```python
from build123d import *

# Parameters (mm, degrees)
SKETCH1_W           = 28.5
SKETCH1_H           = 25
BOSS_EXTRUDE1_DEPTH = 2
SKETCH2_W           = 28.5
SKETCH2_H           = 25
SKETCH2_W_2         = 25.5
SKETCH2_H_2         = 22
BOSS_EXTRUDE2_DEPTH = 10
SKETCH3_W           = 1.5
SKETCH3_H           = 7
CUT_EXTRUDE1_DEPTH  = 10
SKETCH4_W           = 1.5
SKETCH4_H           = 2.5
CUT_EXTRUDE2_DEPTH  = 6
BOSS_EXTRUDE3_DEPTH = 12
CUT_EXTRUDE3_REACH  = 27.348
SKETCH6_R           = 1.75
FILLET1_R           = 1


with BuildPart() as part:
    # Sketch1 → Boss-Extrude1 (new body)
    with BuildSketch(Plane(origin=(0, 0, 0), x_dir=(1, 0, 0), z_dir=(0, 1, 0))):
        Rectangle(SKETCH1_W, SKETCH1_H)
        with BuildLine():
            Line((-9.25, 5), (9.25, 5))
            ThreePointArc((9.25, 5), (9.780330086, 5.219669914), (10, 5.75))
            Line((10, 5.75), (10, 6.25))
            ThreePointArc((10, 6.25), (9.780330086, 6.780330086), (9.25, 7))
            Line((9.25, 7), (-9.25, 7))
            ThreePointArc((-9.25, 7), (-9.780330086, 6.780330086), (-10, 6.25))
            Line((-10, 6.25), (-10, 5.75))
            ThreePointArc((-10, 5.75), (-9.780330086, 5.219669914), (-9.25, 5))
        make_face(mode=Mode.SUBTRACT)
        with BuildLine():
            Line((-9.25, 4), (9.25, 4))
            ThreePointArc((9.25, 4), (9.780330086, 3.780330086), (10, 3.25))
            Line((10, 3.25), (10, 2.75))
            ThreePointArc((10, 2.75), (9.780330086, 2.219669914), (9.25, 2))
            Line((9.25, 2), (-9.25, 2))
            ThreePointArc((-9.25, 2), (-9.780330086, 2.219669914), (-10, 2.75))
            Line((-10, 2.75), (-10, 3.25))
            ThreePointArc((-10, 3.25), (-9.780330086, 3.780330086), (-9.25, 4))
        make_face(mode=Mode.SUBTRACT)
        with BuildLine():
            Line((-9.25, 8), (9.25, 8))
            ThreePointArc((9.25, 8), (9.780330086, 8.219669914), (10, 8.75))
            Line((10, 8.75), (10, 9.25))
            ThreePointArc((10, 9.25), (9.780330086, 9.780330086), (9.25, 10))
            Line((9.25, 10), (-9.25, 10))
            ThreePointArc((-9.25, 10), (-9.780330086, 9.780330086), (-10, 9.25))
            Line((-10, 9.25), (-10, 8.75))
            ThreePointArc((-10, 8.75), (-9.780330086, 8.219669914), (-9.25, 8))
        make_face(mode=Mode.SUBTRACT)
        with BuildLine():
            Line((10, -9.25), (10, -8.75))
            ThreePointArc((10, -8.75), (9.780330086, -8.219669914), (9.25, -8))
            Line((9.25, -8), (-9.25, -8))
            ThreePointArc((-9.25, -8), (-9.780330086, -8.219669914), (-10, -8.75))
            Line((-10, -8.75), (-10, -9.25))
            ThreePointArc((-10, -9.25), (-9.780330086, -9.780330086), (-9.25, -10))
            Line((-9.25, -10), (9.25, -10))
            ThreePointArc((9.25, -10), (9.780330086, -9.780330086), (10, -9.25))
        make_face(mode=Mode.SUBTRACT)
        with BuildLine():
            Line((10, -6.25), (10, -5.75))
            ThreePointArc((10, -5.75), (9.780330086, -5.219669914), (9.25, -5))
            Line((9.25, -5), (-9.25, -5))
            ThreePointArc((-9.25, -5), (-9.780330086, -5.219669914), (-10, -5.75))
            Line((-10, -5.75), (-10, -6.25))
            ThreePointArc((-10, -6.25), (-9.780330086, -6.780330086), (-9.25, -7))
            Line((-9.25, -7), (9.25, -7))
            ThreePointArc((9.25, -7), (9.780330086, -6.780330086), (10, -6.25))
        make_face(mode=Mode.SUBTRACT)
        with BuildLine():
            Line((10, -3.25), (10, -2.75))
            ThreePointArc((10, -2.75), (9.780330086, -2.219669914), (9.25, -2))
            Line((9.25, -2), (-9.25, -2))
            ThreePointArc((-9.25, -2), (-9.780330086, -2.219669914), (-10, -2.75))
            Line((-10, -2.75), (-10, -3.25))
            ThreePointArc((-10, -3.25), (-9.780330086, -3.780330086), (-9.25, -4))
            Line((-9.25, -4), (9.25, -4))
            ThreePointArc((9.25, -4), (9.780330086, -3.780330086), (10, -3.25))
        make_face(mode=Mode.SUBTRACT)
        with BuildLine():
            Line((-10, 0.25), (-10, -0.25))
            ThreePointArc((-10, -0.25), (-9.780330086, -0.780330086), (-9.25, -1))
            Line((-9.25, -1), (9.25, -1))
            ThreePointArc((9.25, -1), (9.780330086, -0.780330086), (10, -0.25))
            Line((10, -0.25), (10, 0.25))
            ThreePointArc((10, 0.25), (9.780330086, 0.780330086), (9.25, 1))
            Line((9.25, 1), (-9.25, 1))
            ThreePointArc((-9.25, 1), (-9.780330086, 0.780330086), (-10, 0.25))
        make_face(mode=Mode.SUBTRACT)
    extrude(amount=BOSS_EXTRUDE1_DEPTH)

    # Sketch2 → Boss-Extrude2 (add)
    with BuildSketch(Plane(origin=(0, 2, 0), x_dir=(1, 0, 0), z_dir=(0, 1, 0))):
        Rectangle(SKETCH2_W, SKETCH2_H)
        Rectangle(SKETCH2_W_2, SKETCH2_H_2, mode=Mode.SUBTRACT)
    extrude(amount=BOSS_EXTRUDE2_DEPTH)

    # Sketch3 → Cut-Extrude1 (cut)
    with BuildSketch(Plane(origin=(0, 12, 0), x_dir=(1, 0, 0), z_dir=(0, 1, 0))):
        with Locations((-13.5, 7.5)):
            Rectangle(SKETCH3_W, SKETCH3_H)
        with Locations((13.5, 7.5)):
            Rectangle(SKETCH3_W, SKETCH3_H)
    extrude(amount=-CUT_EXTRUDE1_DEPTH, mode=Mode.SUBTRACT)

    # Sketch4 → Cut-Extrude2 (cut)
    with BuildSketch(Plane(origin=(0, 12, 0), x_dir=(1, 0, 0), z_dir=(0, 1, 0))):
        with Locations((-13.5, -2)):
            Rectangle(SKETCH4_W, SKETCH4_H)
    extrude(amount=-CUT_EXTRUDE2_DEPTH, mode=Mode.SUBTRACT)

    # Sketch5 → Boss-Extrude3 (add)
    with BuildSketch(Plane.XZ):
        with BuildLine():
            Line((-17.468529919, -4), (-14.25, -4))
            Line((-14.25, -4), (-14.25, 0.75))
            Line((-14.25, 0.75), (-17.468529919, 0.75))
            ThreePointArc((-17.468529919, 0.75), (-18.5, -1.625), (-17.468529919, -4))
        make_face()
        with BuildLine():
            Line((14.25, 0.75), (14.25, -4))
            Line((14.25, -4), (17.468529919, -4))
            ThreePointArc((17.468529919, -4), (18.5, -1.625), (17.468529919, 0.75))
            Line((17.468529919, 0.75), (14.25, 0.75))
        make_face()
    extrude(amount=-BOSS_EXTRUDE3_DEPTH)

    # Sketch6 → Cut-Extrude3 (cut, up to next)
    with BuildSketch(Plane.XZ, mode=Mode.PRIVATE) as cut_extrude3_sk1:
        with Locations(Location((-15.25, -1.625, 0), (0, 0, 270))):
            Circle(SKETCH6_R)
    cut_extrude3_tool1 = extrude(cut_extrude3_sk1.sketch, amount=-CUT_EXTRUDE3_REACH, mode=Mode.PRIVATE) & part.part
    # Sketch6 → Cut-Extrude3 (cut, up to next)
    with BuildSketch(Plane.XZ, mode=Mode.PRIVATE) as cut_extrude3_sk2:
        with Locations(Location((15.25, -1.625, 0), (0, 0, 90))):
            Circle(SKETCH6_R)
    cut_extrude3_tool2 = extrude(cut_extrude3_sk2.sketch, amount=-CUT_EXTRUDE3_REACH, mode=Mode.PRIVATE) & part.part
    add(cut_extrude3_tool1.solids().sort_by_distance((-15.25, 0, -1.625))[0], mode=Mode.SUBTRACT)
    add(cut_extrude3_tool2.solids().sort_by_distance((15.25, 0, -1.625))[0], mode=Mode.SUBTRACT)

    # Fillet1
    fillet1_edges = [part.edges().sort_by_distance(p)[0] for p in [
        (-14.25, 1, -4),
        (14.25, 1, -4),
        (-14.25, 3, 0.75),
        (14.25, 6, 0.75),
        (-13.5, 6, 0.75),
        (-13.5, 6, 3.25),
        (13.5, 2, -4),
        (-13.5, 2, -4),
        (0, 2, -11),
    ]]
    fillet(fillet1_edges, radius=FILLET1_R - 0.0001)  # a hair under: the kernel refuses the full size


solid = part.part
```
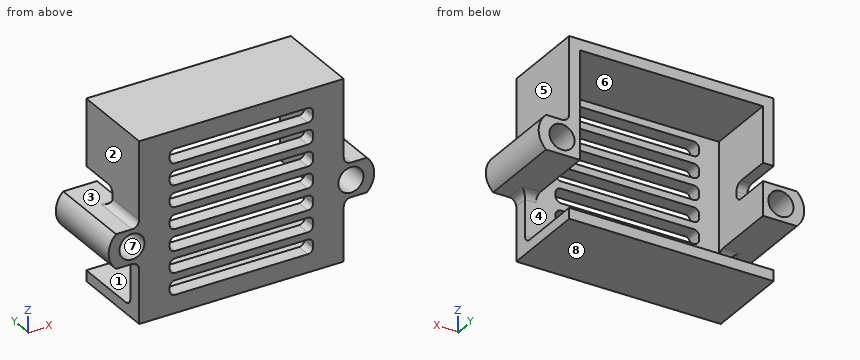
Can you work these out from the model? Positions are in its coordinate system, mm. Face numbers are marked on the shaded views. A direction names the side the tool comes from. Round coordinates to 2 decimals unless told otherwise and drop trailing zeros. Order: outer loops, then holes, each group sorted by start corner. A loop starts at its lowest first (then second) coordinate and runs counter-clockwise, first axis right, second up. Notation, with made-up numbers: (18.5, 22.25) -> (52.5, 22.25) arc R26 ccw to (52.5, 54.25) -> close; hole circle Ø7 at (82, -9). An arc over 180 degrees is marked (long way). Return JSON: item names as keys, results as strings. Group by question number.
1. If we section it at A-A, the plane y = 9.25: Write out the boundary of the cut face in (x, z) (3 decimals), then the cut area to 3 significant figures.
2. I need wall thicknesses on line 1 (X direction, y = 9.5, z = -1.5); line 2 (Z direction, x = -6.5, y = 11); line 3 (X direction, y = 6.5, z = 10.5). Which ranges of each line are inside material? Lowest first, please. Write a range as [from, to].
3. Will these pins go through, and if not, where does the flat tip stop? pin 1 (1.8 mm diameter, centred on x = 17, y = 8, fed in from +Z); pin 2 (6 mm diameter, centred on y = 6.5, z = -5, fed in from -X); pin 3 (3 mm diameter, centred on x = -15.25, z = -1.625, fed in from -Y); pin 4 (2 mm diameter, centred on y = 5, z = 5, fed in from +X).
4. We'd pull the mould along Z, two halves only. Please class the marked faces 5, 6, 7 and 8: released by +Z, released by -Z, zero draft, split by the parting line, or undercut.
5. If we section it at B-B, the plane y = 4.5: Write out the boundary of the cut face in (x, z) (3 decimals), then the cut area to 3 significant figures.
6. If we section it at D-D, the plane x = 6: Count the separate pieces of the cut face and the enclosed holes in it, then the cut area to 3 significant figures.
7. If we section it at C-C, the plane z = -1.5: Write out the boundary of the cut face in (x, y), then the cut area to 3 significant figures.
8. Which directions (+Z, -Z, +X, -X, +Y, -Y) give clear straight access to the entire face, cutting with the end or side of a thin tool? Please do the marked faces 1, 2, 3 and 4.
Output values:
{
 "1": {"outline": "(-17.469, -4) -> (-12.75, -4) -> (-12.75, 0.75) -> (-17.469, 0.75) arc R3.25 ccw to start; (-14.25, -12.5) -> (14.25, -12.5) -> (14.25, -11) -> (-14.25, -11) -> close; (-14.25, 3.25) -> (-12.75, 3.25) -> (-12.75, 11) -> (12.75, 11) -> (12.75, -4) -> (17.469, -4) arc R3.25 ccw to (17.469, 0.75) -> (15.25, 0.75) arc R1 cw to (14.25, 1.75) -> (14.25, 12.5) -> (-14.25, 12.5) -> close; hole circle Ø3.5 at (-15.25, -1.625); hole circle Ø3.5 at (15.25, -1.625)", "area": "145 mm²"},
 "2": {"line 1": "[-18.5, -17], [-13.5, -12.75], [12.75, 13.5], [17, 18.5]", "line 2": "[-12.5, -11], [11, 12.5]", "line 3": "[-14.25, -12.75], [12.75, 14.25]"},
 "3": {"pin 1": "z = 0.75", "pin 2": "x = -18.48", "pin 3": "through", "pin 4": "x = 14.25"},
 "4": {"face 5": "zero draft", "face 6": "undercut", "face 7": "undercut", "face 8": "released by -Z"},
 "5": {"outline": "(-17.469, -4) -> (-12.75, -4) -> (-12.75, 11) -> (12.75, 11) -> (12.75, -4) -> (17.469, -4) arc R3.25 ccw to (17.469, 0.75) -> (15.25, 0.75) arc R1 cw to (14.25, 1.75) -> (14.25, 12.5) -> (-14.25, 12.5) -> (-14.25, 1.75) arc R1 cw to (-15.25, 0.75) -> (-17.469, 0.75) arc R3.25 ccw to start; (-14.25, -12.5) -> (14.25, -12.5) -> (14.25, -11) -> (-14.25, -11) -> close; hole circle Ø3.5 at (-15.25, -1.625); hole circle Ø3.5 at (15.25, -1.625)", "area": "149 mm²"},
 "6": {"separate pieces": "8", "enclosed holes": "0", "area": "52.2 mm²"},
 "7": {"outline": "(-18.5, 0) -> (-17, 0) -> (-17, 12) -> (-18.5, 12) -> close; (-13.5, 0) -> (13.5, 0) -> (13.5, 12) -> (12.75, 12) -> (12.75, 2) -> (-12.75, 2) -> (-12.75, 12) -> (-13.5, 12) -> close; (17, 0) -> (18.5, 0) -> (18.5, 12) -> (17, 12) -> close", "area": "105 mm²"},
 "8": {"face 1": "+X, -X, +Y", "face 2": "+Z, -X, +Y, -Y", "face 3": "-X, +Y", "face 4": "+Y"}
}
